Could you check a few things on this drawing? It's one solid part, dimensions in mm from its lowest x, y, z. Round coordinates to 2 decimals unless told otherwise and drop trailing zeros. Order: outer loops, then holes, each group sorted by start corner. A loop starts at its lowest first (then second) coordinate and runs counter-clockwise, first axis right, second up. Notation, with made-up numbers: (1.25, 87.25) -> (20.25, 87.25) arc R15 cw to (20.25, 94.25) -> close; hole circle Ø9 at (80.25, 63). An arc over 180 degrees is marked (long way). Use a Markdown table: item, result. Add a question column.
(1) I'm going to push flat-ended pins straight in: P1, Ø2, axis at x = 10.5, z = 16, coming from the +Y side; P2, Ø1.2, axis at y = 3, z = 18.5, coming from the -X side; P3, Ø3.5, axis at x = 17, z = 6.5, coming from the +Y side; P4, Ø0.8, axis at y = 3, z = 19, coming from the +X side. Where does each tip first touch, or does it pass through?
(2) Thinking about a two-plate mould opening in X: for the marked faces 1, 2, 3 and 4, which applies, pulls with the +X half, pulls with the -X half, needs draft (parallel to the pull), parting line crosses it, or undercut?
(3) If I drill on probe 1 along X at (y, z) = (1, 4.5); probe 2 along X at (y, z) = (2.3, 10.25); probe 3 along Z at (x, y) = (15, 0.85), over which ranges is the centre line in solid material (lowest first)?
(4) I want a section at B-B, the plane z = 4.5. Please give me the cut outline in (x, y), then the cut area to 3 significant figures.
(5) I want a section at D-D, the plane z = 17. Please give me the cut outline in (x, y).
(6) I want a section at A-A, the plane x = 19.5. Please give me the cut outline in (y, z), then the cut area to 3 significant figures.
(7) I want a section at C-C, the plane y = 1.8. Please give me the cut outline in (x, z), then the cut area to 3 significant figures.
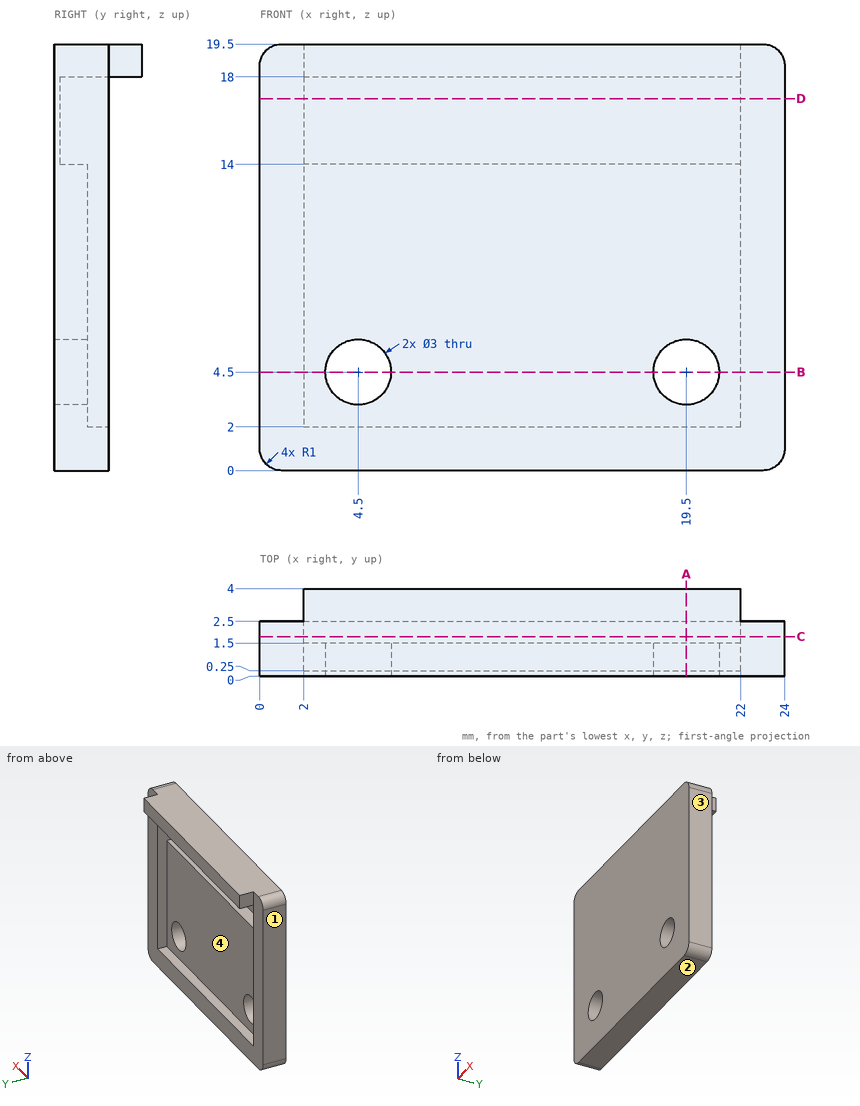
Taken from the geometry:
| question | item | result |
|---|---|---|
| 1 | P1 | stops at y = 0.25 |
| 1 | P2 | stops at x = 0 |
| 1 | P3 | stops at y = 1.5 |
| 1 | P4 | stops at x = 22 |
| 2 | face 1 | pulls with the -X half |
| 2 | face 2 | needs draft |
| 2 | face 3 | pulls with the +X half |
| 2 | face 4 | undercut |
| 3 | probe 1 | x = 0 to 3, 6 to 18, 21 to 24 |
| 3 | probe 2 | x = 0 to 2, 22 to 24 |
| 3 | probe 3 | z = 0 to 14, 18 to 19.5 |
| 4 | outline | (0, 0) -> (3, 0) -> (3, 1.5) -> (2, 1.5) -> (2, 2.5) -> (0, 2.5) -> close; (6, 0) -> (18, 0) -> (18, 1.5) -> (6, 1.5) -> close; (21, 0) -> (24, 0) -> (24, 2.5) -> (22, 2.5) -> (22, 1.5) -> (21, 1.5) -> close |
| 4 | area | 31.0 mm2 |
| 5 | outline | (0, 0) -> (24, 0) -> (24, 2.5) -> (22, 2.5) -> (22, 0.25) -> (2, 0.25) -> (2, 2.5) -> (0, 2.5) -> close |
| 6 | outline | (0, 0) -> (2.5, 0) -> (2.5, 2) -> (1.5, 2) -> (1.5, 3) -> (0, 3) -> close; (0, 6) -> (1.5, 6) -> (1.5, 14) -> (0.25, 14) -> (0.25, 18) -> (4, 18) -> (4, 19.5) -> (0, 19.5) -> close |
| 6 | area | 25.5 mm2 |
| 7 | outline | (0, 1) arc R1 ccw to (1, 0) -> (23, 0) arc R1 ccw to (24, 1) -> (24, 18.5) arc R1 ccw to (23, 19.5) -> (1, 19.5) arc R1 ccw to (0, 18.5) -> close; hole (2, 2) -> (22, 2) -> (22, 18) -> (2, 18) -> close |
| 7 | area | 147 mm2 |
